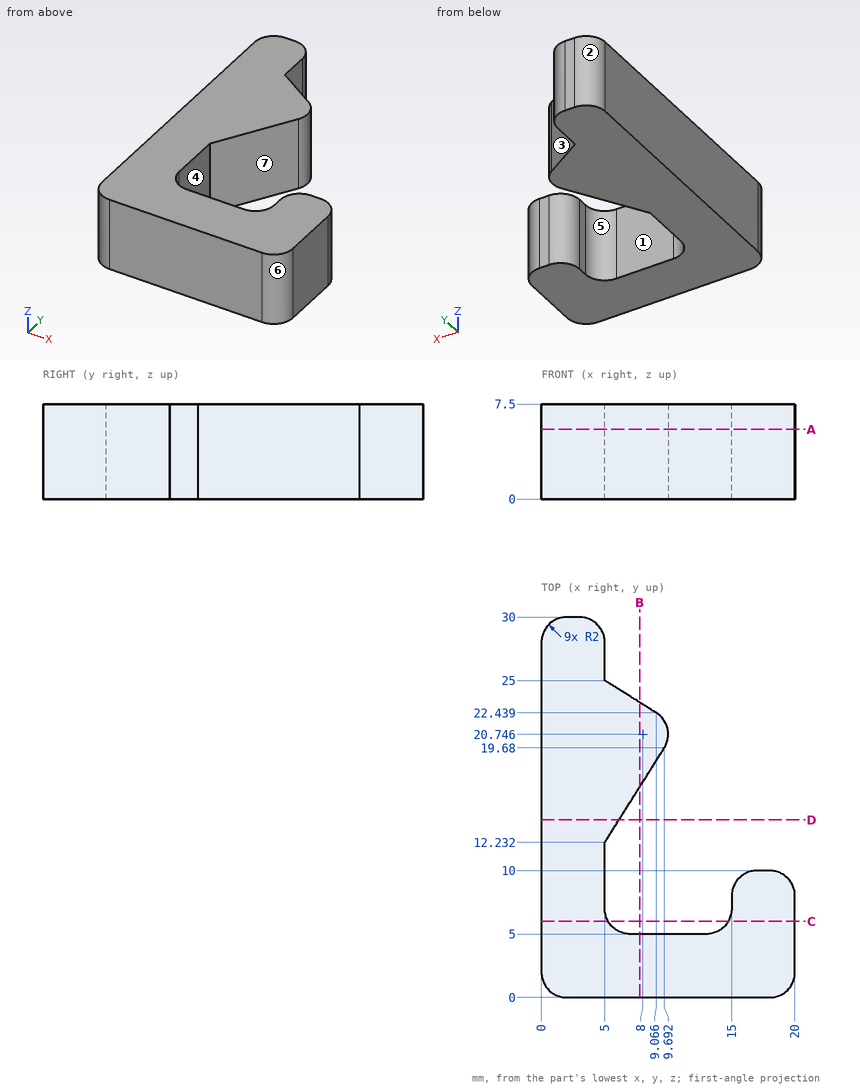
Drawing for the job (mm, zero at the part's lowest x, y, z). A direction names the side the tool comes from. Round coordinates to 2 decimals unless told otherwise and drop trailing zeros. Write each loop counter-clockwise with the first axis right and the second up, starting at its lowest first coordinate (ties: lowest second). Pieces come first, ordered by that corner, then holes. Notation, with made-up numbers: (0, -22.5) - (17, -22.5) arc R26 cw to (17, -3.5) - close; hole circle Ø11 at (-8, -13.5). An arc over 180 degrees is marked (long way). Return JSON: item names as keys, results as strings. Group by question number.
Item 1: Band-saw the part on D-D on y = 14. List the corners of the cut face in (x, z).
Item 2: Band-saw the part on A-A on z = 5.5. List the corners of the cut face in (x, y).
Item 3: Band-saw the part on C-C on y = 6. List the corners of the cut face in (x, z).
Item 4: Band-saw the part on B-B on x = 7.75. List the corners of the cut face in (y, z).
Item 5: Mould opens along X. For the marked faces 1, 2 and 3 say: +X half, -X half, draft (parallel to the pull), parting line (faces both ways), or undercut.
Item 6: Flat gauge pins, fed straight in: pin 1 Ø1.8 at (x, z) = (9, 2.5) entering from +Y; pin 2 Ø12 at (x, y) = (11, 6.5) entering from -Z; pin 3 Ø3.5 at (y, z) = (26, 4) entering from +X. Where does each tip first touch, or does it go through?
Item 7: Probe probe 1 along X at (y, z) = (25.5, 5.5); probe 2 along Y at (x, z) = (7.75, 6.5) (1 decimal); probe 3 along Y at (x, z) = (17.25, 1.25). List the from-to ranges inside material, lowest first.
Item 8: 3-axis set-ups, long thin cutter, end or side, ignore diameter. For the marked faces 4, 5, 6 and 7: which of +Z, -Z, +X, -X, +Y, -Y reach the whole face in a straight line?
Resolved:
{
 "1": {"outline": "(0, 0) - (6.11, 0) - (6.11, 7.5) - (0, 7.5) - close"},
 "2": {"outline": "(0, 2) arc R2 ccw to (2, 0) - (18, 0) arc R2 ccw to (20, 2) - (20, 8) arc R2 ccw to (18, 10) - (17, 10) arc R2 ccw to (15, 8) - (15, 7) arc R2 cw to (13, 5) - (7, 5) arc R2 cw to (5, 7) - (5, 12.23) - (9.69, 19.68) arc R2 ccw to (9.07, 22.44) - (5, 25) - (5, 28) arc R2 ccw to (3, 30) - (2, 30) arc R2 ccw to (0, 28) - close"},
 "3": {"outline": "(0, 0) - (5.27, 0) - (5.27, 7.5) - (0, 7.5) - close; (14.73, 0) - (20, 0) - (20, 7.5) - (14.73, 7.5) - close"},
 "4": {"outline": "(0, 0) - (5, 0) - (5, 7.5) - (0, 7.5) - close; (16.6, 0) - (23.27, 0) - (23.27, 7.5) - (16.6, 7.5) - close"},
 "5": {"face 1": "undercut", "face 2": "-X half", "face 3": "+X half"},
 "6": {"pin 1": "stops at y = 23.05", "pin 2": "stops at z = 0", "pin 3": "stops at x = 6.19"},
 "7": {"probe 1": "x = 0 to 5", "probe 2": "y = 0 to 5, 16.6 to 23.3", "probe 3": "y = 0 to 10"},
 "8": {"face 4": "+Z, -Z", "face 5": "+Z, -Z, +Y", "face 6": "+Z, -Z, +X, -Y", "face 7": "+Z, -Z, +X"}
}
